```python
from build123d import *

# Parameters (mm, degrees)
SKETCH1_R           = 1.9
BOSS_EXTRUDE1_DEPTH = 19.4
SKETCH2_R           = 4
BOSS_EXTRUDE2_DEPTH = 2
CHAMFER1_SIZE       = 0.5
SKETCH3_R           = 1
CUT_EXTRUDE1_DEPTH  = 3


with BuildPart() as part:
    # Sketch1 → Boss-Extrude1 (new body)
    with BuildSketch(Plane(origin=(0, 0, 0), x_dir=(1, 0, 0), z_dir=(0, 1, 0))):
        with Locations(Location((0, 0, 0), (0, 0, 270))):
            Circle(SKETCH1_R)
    extrude(amount=BOSS_EXTRUDE1_DEPTH)

    # Sketch2 → Boss-Extrude2 (add)
    with BuildSketch(Plane.XZ):
        with Locations(Location((0, 0, 0), (0, 0, 270))):
            Circle(SKETCH2_R)
    extrude(amount=BOSS_EXTRUDE2_DEPTH)

    # Chamfer1
    chamfer1_edges = [part.edges().sort_by_distance(p)[0] for p in [
        (0, -2, 4),
    ]]
    chamfer(chamfer1_edges, length=CHAMFER1_SIZE)

    # Sketch3 → Cut-Extrude1 (cut)
    with BuildSketch(Plane(origin=(0, 19.4, 0), x_dir=(1, 0, 0), z_dir=(0, 1, 0))):
        with Locations(Location((0, 0, 0), (0, 0, 270))):
            Circle(SKETCH3_R)
    extrude(amount=-CUT_EXTRUDE1_DEPTH, mode=Mode.SUBTRACT)


solid = part.part
```
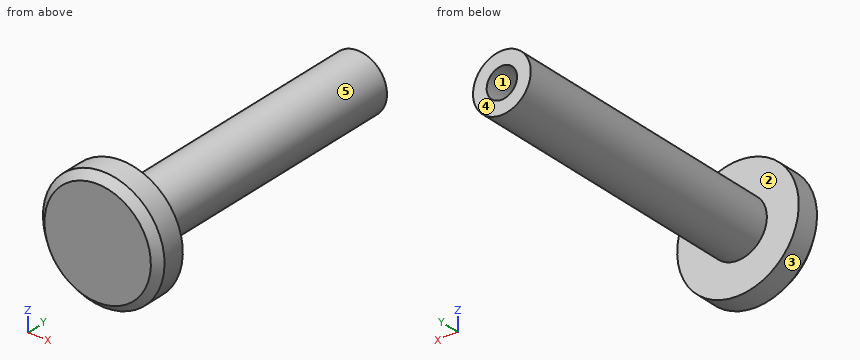
Model file for the job. Use its own axes, mm. Face numbers are marked on the shaded views. A direction names the side the tool comes from. Coordinates: 2 decimals unless noted, no trailing zeros. Loops run counter-clockwise (first coordinate to the right, second up) from the corner with the lowest first, then second, coordinate; pieces in that order, holes last. Notation, with made-up numbers: (85, 34.5) - (103, 34.5) arc R14 ccw to (103, 54.5) - close; hole circle Ø3 at (31.25, 75.25). An arc over 180 degrees is marked (long way). Answer as a JSON object with one key per item and string values. Group by question number.
(1) Cut at A-A (x = 0). Give the cut face in (y, z).
(2) Cut at B-B (z = 0). Give the cut face in (x, y), then the cut area to 3 significant figures.
(3) Flat gauge pins, fed straight in: pin 1 (3 mm diameter, centred on y = 7.5, z = 2.5, fed in from -X); pin 2 (1 mm diameter, centred on x = -2.5, z = 1, fed in from +Y); pin 3 (4 mm diameter, centred on x = -2, y = 10.5, fed in from +Z). Where does each tip first touch, or does it go through?
(4) Two-plate mould, pull along Z, no slides. Class the marked faces 1, 2 and 3: released by +Z, released by -Z, zero draft, split by the parting line, or undercut.
(5) Tool access for the marked faces 4 and 5: list every direction of +Z, -Z, +X, -X, +Y, -Y with a clear straight run to the whole face (end or side of a thin tool).
(6) Cut at C-C (y = 6.5). Give the cut face in (x, z), then the cut area to 3 significant figures.
(7) Probe line 1 along X through (y, z) = (18.1, 0); line 2 along Y through (x, z) = (-1.75, -1.5); line 3 along Y through (x, z) = (-0.25, 0). List the from-to ranges inside material, lowest first.
Geometry says:
{
 "1": {"outline": "(-2, -3.5) - (-1.5, -4) - (0, -4) - (0, -1.9) - (19.4, -1.9) - (19.4, -1) - (16.4, -1) - (16.4, 1) - (19.4, 1) - (19.4, 1.9) - (0, 1.9) - (0, 4) - (-1.5, 4) - (-2, 3.5) - close"},
 "2": {"outline": "(-4, -1.5) - (-3.5, -2) - (3.5, -2) - (4, -1.5) - (4, 0) - (1.9, 0) - (1.9, 19.4) - (1, 19.4) - (1, 16.4) - (-1, 16.4) - (-1, 19.4) - (-1.9, 19.4) - (-1.9, 0) - (-4, 0) - close", "area": "83.5 mm^2"},
 "3": {"pin 1": "stops at x = -1.62", "pin 2": "stops at y = 0", "pin 3": "stops at z = 1.9"},
 "4": {"face 1": "undercut", "face 2": "zero draft", "face 3": "split by the parting line"},
 "5": {"face 4": "+Z, -Z, +X, -X, +Y", "face 5": "+Y"},
 "6": {"outline": "circle Ø3.8 at (0, 0)", "area": "11.3 mm^2"},
 "7": {"line 1": "x = -1.9 to -1, 1 to 1.9", "line 2": "y = -2 to 0", "line 3": "y = -2 to 16.4"}
}
